The drawing under review shows one solid part. Ordinate dimensions are in mm from its lowest x, y, z. Give positions to 0.01 mm unless a question says otherwise; leave off trailing zeros. Order: outer loops, then holes, each group sorted by start corner. A loop starts at its lowest first (then second) coordinate and runs counter-clockwise, first axis right, second up. Notation, with made-up numbers: (74, -14) - (105, -14) arc R23 ccw to (105, -1) - close; hole circle Ø9 at (74, 58.25). An arc over 180 degrees is marked (long way). Use CSV: the item, a comma, the result in double quotes. Start each with the question number.
1. Take a section at B-B, the plane y = 4. State the section outline as (x, z) points, then the cut area to 3 significant figures.
2. Take a section at C-C, the plane x = 9. State the section outline as (y, z) points, then the cut area to 4 significant figures.
3. Take a section at D-D, the plane y = 9.5. State the section outline as (x, z) points, then the cut area to 3 significant figures.
4. For pin 1 (1.6 mm diameter, centred on y = 6, z = 5.5, fed in from -X); pin 2 (1 mm diameter, centred on x = 58, y = 7.5, fed in from -Z); pin 3 (4 mm diameter, centred on y = 8.5, z = 3.5, fed in from -X), all flat-tipped, find the tip position at first contact; note any pin that passes through.
5. Draft analysis for pull direction X (two halves, no side actions). For the marked faces 1, 2 and 3, state which applies: released by +X, released by -X, zero draft, split by the parting line, or undercut.
6. To check wall thickness, follow line 1 (X direction, y = 10.25, z = 3.5); line 2 (Z direction, x = 48.5, y = 1.75); line 3 (X direction, y = 7.25, z = 1.5). State the ranges of each line that lie inside material, in increasing order. Write a range as [from, to].
7. Take a section at A-A, the plane z = 4.25. State the section outline as (x, y) points, then the cut area to 3 significant figures.
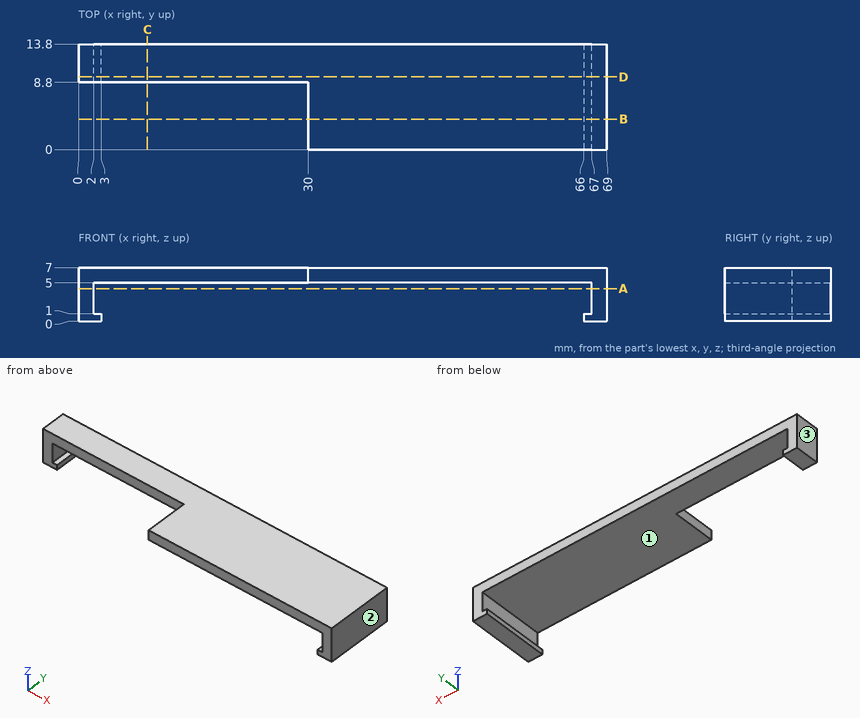
Determined:
1,outline,"(30, 5) - (67, 5) - (67, 1) - (66, 1) - (66, 0) - (69, 0) - (69, 7) - (30, 7) - close"
1,area,"89.0 mm²"
2,outline,"(8.8, 5) - (13.8, 5) - (13.8, 7) - (8.8, 7) - close"
2,area,"10.00 mm²"
3,outline,"(0, 0) - (3, 0) - (3, 1) - (2, 1) - (2, 5) - (67, 5) - (67, 1) - (66, 1) - (66, 0) - (69, 0) - (69, 7) - (0, 7) - close"
3,area,"160 mm²"
4,pin 1,"stops at x = 30"
4,pin 2,"stops at z = 5"
4,pin 3,"stops at x = 0"
5,face 1,"undercut"
5,face 2,"released by +X"
5,face 3,"released by -X"
6,line 1,"x = [0, 2], [67, 69]"
6,line 2,"z = [5, 7]"
6,line 3,"x = [67, 69]"
7,outline,"(0, 8.8) - (2, 8.8) - (2, 13.8) - (0, 13.8) - close; (67, 0) - (69, 0) - (69, 13.8) - (67, 13.8) - close"
7,area,"37.6 mm²"
